from build123d import *
from build123d.topology import SkipClean

# Parameters (mm, degrees)
SKETCH3_W           = 9.65
SKETCH3_H           = 18.81667
SKETCH3_W_2         = 7.65
SKETCH3_H_2         = 16.81667
EXTRUDE_THIN1_DEPTH = 2.5
BOSS_EXTRUDE2_DEPTH = 2.5
CUT_EXTRUDE1_DEPTH  = 2.5
FILLET1_R           = 4


with BuildPart() as part:
    # Sketch3 → Extrude-Thin1 (new body)
    with BuildSketch(Plane.XY):
        with Locations((10.605490461, -24)):
            Rectangle(SKETCH3_W, SKETCH3_H)
        with Locations((10.605490461, -24)):
            Rectangle(SKETCH3_W_2, SKETCH3_H_2, mode=Mode.SUBTRACT)
    extrude(amount=EXTRUDE_THIN1_DEPTH)

    # Sketch4 → Boss-Extrude2 (add)
    with BuildSketch(Plane.XY.offset(2.5)):
        with BuildLine():
            ThreePointArc((5.780490461, -15.591665), (5.07338368, -13.884558219), (6.780490461, -14.591665))
            Line((6.780490461, -14.591665), (6.917868383, -14.591665))
            ThreePointArc((6.917868383, -14.591665), (6.979465006, -14.329673307), (7.000160375, -14.061334914))
            ThreePointArc((7.000160375, -14.061334914), (3.837613447, -13.02827578), (5.780490461, -15.729042922))
            Line((5.780490461, -15.729042922), (5.780490461, -15.591665))
        make_face()
        with BuildLine():
            ThreePointArc((17.710820547, -33.938665086), (16.993879681, -32.526118157), (15.430490461, -32.270957078))
            Line((15.430490461, -32.270957078), (15.430490461, -32.408335))
            ThreePointArc((15.430490461, -32.408335), (16.137597242, -32.701228219), (16.430490461, -33.408335))
            ThreePointArc((16.430490461, -33.408335), (15.430490461, -34.408335), (14.430490461, -33.408335))
            Line((14.430490461, -33.408335), (14.293112539, -33.408335))
            ThreePointArc((14.293112539, -33.408335), (15.692482154, -35.667969717), (17.710820547, -33.938665086))
        make_face()
    extrude(amount=-BOSS_EXTRUDE2_DEPTH)

    # Sketch4<2> → Cut-Extrude1 (cut)
    with SkipClean():  # the faces are left unmerged after this step: merging them gives an invalid solid
        with BuildSketch(Plane.XY.offset(2.5)):
            with BuildLine():
                Line((5.780490461, -14.591665), (6.780490461, -14.591665))
                ThreePointArc((6.780490461, -14.591665), (5.07338368, -13.884558219), (5.780490461, -15.591665))
                Line((5.780490461, -15.591665), (5.780490461, -14.591665))
            make_face()
            with BuildLine():
                ThreePointArc((6.487597245, -15.298771778), (6.704369994, -14.97434843), (6.780490461, -14.591665))
                Line((6.780490461, -14.591665), (5.780490461, -14.591665))
                Line((5.780490461, -14.591665), (5.780490461, -15.591665))
                ThreePointArc((5.780490461, -15.591665), (6.163173895, -15.515544532), (6.487597245, -15.298771778))
            make_face()
            with BuildLine():
                ThreePointArc((15.430490461, -32.408335), (15.047807029, -32.484455467), (14.72338368, -32.701228219))
                ThreePointArc((14.72338368, -32.701228219), (14.506610928, -33.025651568), (14.430490461, -33.408335))
                Line((14.430490461, -33.408335), (15.430490461, -33.408335))
                Line((15.430490461, -33.408335), (15.430490461, -32.408335))
            make_face()
            with BuildLine():
                ThreePointArc((16.430490461, -33.408335), (16.137597242, -32.701228219), (15.430490461, -32.408335))
                Line((15.430490461, -32.408335), (15.430490461, -33.408335))
                Line((15.430490461, -33.408335), (14.430490461, -33.408335))
                ThreePointArc((14.430490461, -33.408335), (15.430490461, -34.408335), (16.430490461, -33.408335))
            make_face()
        extrude(amount=-CUT_EXTRUDE1_DEPTH, mode=Mode.SUBTRACT)

    # Fillet1
    fillet1_edges = [part.edges().sort_by_distance(p)[0] for p in [
        (6.917868383, -14.591665, 1.25),
        (5.780490461, -15.729042922, 1.25),
        (14.293112539, -33.408335, 1.25),
        (15.430490461, -32.270957078, 1.25),
    ]]
    fillet(fillet1_edges, radius=FILLET1_R)


solid = part.part
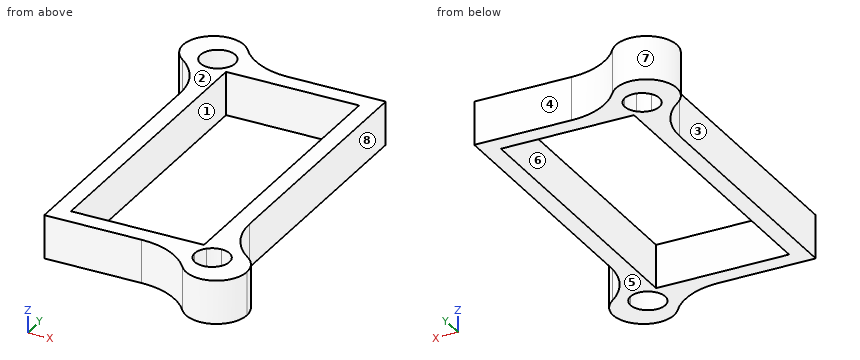
Geometry: final body of the model. Coordinates: model frame, mm. Face numbers are marked on the shaded views. A direction names the side the tool comes from. Give positions to 0.01 mm unless a question says otherwise; leave off trailing zeros. Loops run counter-clockwise (first coordinate to the right, second up) from the corner with the lowest first, then second, coordinate; pieces in that order, holes last. Notation, with made-up numbers: (-18, 33.5) - (38, 33.5) arc R28 cw to (38, 70.5) - close; hole circle Ø9 at (3, 38.25). An arc over 180 degrees is marked (long way). One line per question, with ' | ' between items. Start each with the question number.
(1) Section query C-C on z = 1.8. Count the separate pieces of the cut face and the enclosed holes in it, then the cut area to 3 significant figures.
(2) Contact query for flat-ended pins moving along their axis: pin 1 (2 mm diameter, centred on x = 7.5, y = -17.5, fed in from -Z); pin 2 (0.8 mm diameter, centred on y = -20, z = 1.5, fed in from +X); pin 3 (1.2 mm diameter, centred on y = -25, z = 2, fed in from -X); pin 4 (0.8 mm diameter, centred on x = 12.5, z = 1.5, fed in from -Y). Output: stop coordinate, or through.
(3) Section query B-B on x = 12.25. Return loops of the section in (y, z).
(4) Ray query, line 1 (X direction, y = -25.5, z = 0.2); line 2 (X direction, y = -32, z = 0.65); line 3 (Y direction, x = 16, z = 0.2). Return the intervals inside material, ascending. Write a range as from..to.
(5) Reachability of the marked faces 1, 2, 3, 4 and 5 from +Z, -Z, +X, -X, +Y, -Y: full face, straight path, thin tool, end or side. Return the list, or none.
(6) Section query A-A on y = -24.75. Return loops of the section in (x, z).
(7) Pull-direction query (Y, two-part tool) for the marked faces 6, 7 and 8; classes: released by +Y, released by -Y, zero draft, split by the parting line, or undercut.
The answers:
1) separate pieces: 1 | enclosed holes: 3 | area: 68.6 mm2
2) pin 1: z = 0 | pin 2: x = 15.43 | pin 3: x = 5.78 | pin 4: y = -33.71
3) outline: (-33.51, 0) - (-32.41, 0) - (-32.41, 2.5) - (-33.51, 2.5) - close; (-15.59, 0) - (-14.59, 0) - (-14.59, 2.5) - (-15.59, 2.5) - close
4) line 1: 5.78..6.78, 14.43..15.43 | line 2: 5.78..6.78, 14.43..16.43 | line 3: -35.69..-34.23, -32.59..-31.41
5) face 1: +Z, -Z | face 2: +Z, +X, -X, +Y, -Y | face 3: +Z, -Z, -X, -Y | face 4: +Z, -Z, +X, +Y | face 5: -Z, +X, -X, +Y, -Y
6) outline: (5.78, 0) - (6.78, 0) - (6.78, 2.5) - (5.78, 2.5) - close; (14.43, 0) - (15.43, 0) - (15.43, 2.5) - (14.43, 2.5) - close
7) face 6: undercut | face 7: split by the parting line | face 8: zero draft
